```python
from build123d import *

# Parameters (mm, degrees)
ESQUISSE1_R        = 24.5
ESQUISSE1_R_2      = 1.5
ESQUISSE1_R_3      = 6.3
BOSS_EXTRU_1_DEPTH = 16
CHANFREIN1_SIZE    = 1


with BuildPart() as part:
    # Esquisse1 → Boss.-Extru.1 (new body)
    with BuildSketch(Plane(origin=(0, 0, 0), x_dir=(1, 0, 0), z_dir=(0, 1, 0))):
        Circle(ESQUISSE1_R)
        with Locations((0, 12.5)):
            Circle(ESQUISSE1_R_2, mode=Mode.SUBTRACT)
        with Locations((12.5, 0)):
            Circle(ESQUISSE1_R_2, mode=Mode.SUBTRACT)
        with Locations((0, -12.5)):
            Circle(ESQUISSE1_R_2, mode=Mode.SUBTRACT)
        with Locations((-12.5, 0)):
            Circle(ESQUISSE1_R_2, mode=Mode.SUBTRACT)
        with Locations((7.753017526, 7.753017526)):
            Circle(ESQUISSE1_R_2, mode=Mode.SUBTRACT)
        with Locations((7.753017526, -7.753017526)):
            Circle(ESQUISSE1_R_2, mode=Mode.SUBTRACT)
        with Locations((-7.753017526, -7.753017526)):
            Circle(ESQUISSE1_R_2, mode=Mode.SUBTRACT)
        with Locations((-7.753017526, 7.753017526)):
            Circle(ESQUISSE1_R_2, mode=Mode.SUBTRACT)
        Circle(ESQUISSE1_R_3, mode=Mode.SUBTRACT)
    extrude(amount=BOSS_EXTRU_1_DEPTH)

    # Chanfrein1
    chanfrein1_edges = [part.edges().sort_by_distance(p)[0] for p in [
        (-24.5, 16, 0),
    ]]
    chamfer(chanfrein1_edges, length=CHANFREIN1_SIZE)


solid = part.part
```
CAD build for the part. Positions are in the model's coordinates, mm. Give positions to 0.01 mm unless a question says otherwise; leave off trailing zeros. Write each loop counter-clockwise with the first axis right and the second up, starting at its lowest first coordinate (ties: lowest second). Pieces come first, ordered by that corner, then holes. Notation, with made-up numbers: M 28.25,81.5 L 69.25,81.5 A26 ccw 69.25,114.5 Z; hole C 2,57 d5. An arc over 180 degrees is marked long. Return JSON: item names as keys, results as strings. Group by question number.
(1) Mould opens along Z. For faces 1 (the face through (-14, 8, 0)), 2 (the face through (5, 16, 5)), 3 (the face through (13.17, 7.4, -20.66)) say: pulls with the +Z half, pulls with the -Z half, needs draft (parallel to the pull), parting line crosses it, or undercut.
(2) Band-saw the part on A-A (x = 0). Give the cut face in (y, z).
(3) Flat gauge pins, fed straight in: pin 1 Ø1.8 at (x, z) = (7.75, -7.75) entering from -Y; pin 2 Ø4 at (y, z) = (7.5, 19) entering from +X; pin 3 Ø1 at (y, z) = (9, 11) entering from +X; pin 4 Ø6 at (y, z) = (2, -6) entering from -X. Where does each tip first touch, or does it go through?
(4) Drill centre lines: L1, parallel to Z at x = 0, y = 11.5; L2, parallel to Z at x = -0.5, y = 2.5; L3, parallel to X at y = 12.25, z = 12.5. Where is each one in solid material? Low to high. Write a range as [from, to].
(5) Band-saw the part on B-B (z = 0). Give the cut face in (x, y).
(6) Band-saw the part on C-C (y = 8.5). State how many separate pieces and enclosed holes the cut face has, and give its area (3 significant figures).
Entries:
{
 "1": {"face 1": "undercut", "face 2": "needs draft", "face 3": "parting line crosses it"},
 "2": {"outline": "M 0,-24.5 L 15,-24.5 L 16,-23.5 L 16,-14 L 0,-14 Z; M 0,-11 L 16,-11 L 16,-6.3 L 0,-6.3 Z; M 0,6.3 L 16,6.3 L 16,11 L 0,11 Z; M 0,14 L 16,14 L 16,23.5 L 15,24.5 L 0,24.5 Z"},
 "3": {"pin 1": "passes through", "pin 2": "stops at x = 17.64", "pin 3": "stops at x = 22.14", "pin 4": "stops at x = -24.32"},
 "4": {"L1": "z = [-24.5, -14], [-11, -6.3], [6.3, 11], [14, 24.5]", "L2": "z = [-24.49, -13.91], [-11.09, -6.28], [6.28, 11.09], [13.91, 24.49]", "L3": "x = [-21.07, -1.5], [1.5, 21.07]"},
 "5": {"outline": "M -24.5,0 L -14,0 L -14,16 L -23.5,16 L -24.5,15 Z; M -11,0 L -6.3,0 L -6.3,16 L -11,16 Z; M 6.3,0 L 11,0 L 11,16 L 6.3,16 Z; M 14,0 L 24.5,0 L 24.5,15 L 23.5,16 L 14,16 Z"},
 "6": {"separate pieces": "1", "enclosed holes": "9", "area": "1,700 mm^2"}
}
